For this review, use the dimensioned drawing (mm, ordinates from the lowest corner) and the shaded views. A direction names the side the tool comes from. Coordinates: 2 decimals unless noted, no trailing zeros. Write each loop counter-clockwise with the first axis right and the second up, starting at its lowest first coordinate (ties: lowest second). Pieces come first, ordered by that corner, then holes. Notation, with made-up numbers: (-28.5, 55.25) - (-6.5, 55.25) arc R25 cw to (-6.5, 71.25) - close; hole circle Ø9 at (44, 10.25). An arc over 180 degrees is marked (long way). Answer as a JSON object with one key per item and string values.
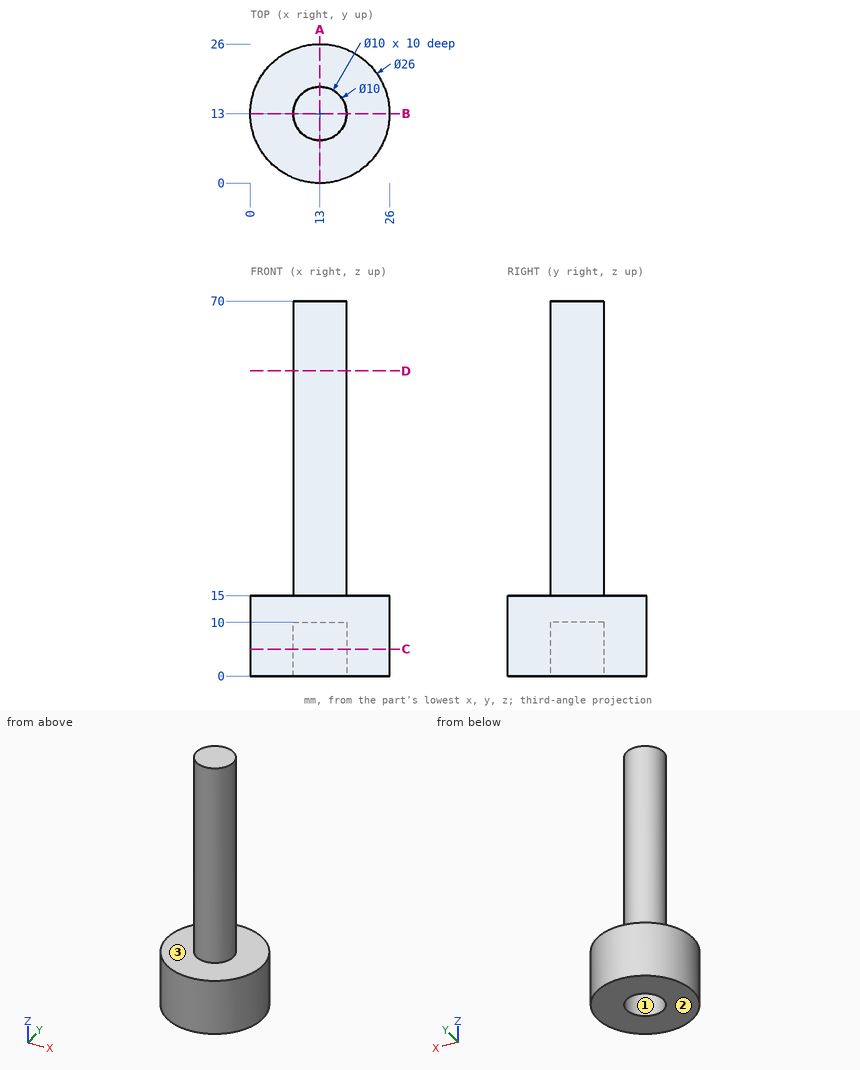
(1) Take a section at C-C, the plane z = 5. Write out the cut boundary in (x, y), and give its area (3 significant figures).
Solved:
{"outline": "circle Ø26 at (13, 13); hole circle Ø10 at (13, 13)", "area": "452 mm^2"}
(2) Take a section at D-D, the plane z = 57. Write out the cut boundary in (x, y), and give its area (3 significant figures).
Solved:
{"outline": "circle Ø10 at (13, 13)", "area": "78.5 mm^2"}
(3) To check wall thickness, follow line 1 (Y direction, x = 13, z = 5.75); line 2 (Z direction, x = 22, y = 4.75); line 3 (Y direction, x = 12.75, z = 16.5). State the ranges of each line that lie inside material, in increasing order. Write a range as from..to.
Solved:
{"line 1": "y = 0..8, 18..26", "line 2": "z = 0..15", "line 3": "y = 8.01..17.99"}
(4) Take a section at A-A, the plane x = 13. Write out the cut boundary in (y, z), and give its area (3 significant figures).
Solved:
{"outline": "(0, 0) - (8, 0) - (8, 10) - (18, 10) - (18, 0) - (26, 0) - (26, 15) - (18, 15) - (18, 70) - (8, 70) - (8, 15) - (0, 15) - close", "area": "840 mm^2"}
(5) Tool access review of the marked faces 1, 2 and 3: name each direction out of +Z, -Z, +X, -X, +Y, -Y from which nothing blocks a thin tool from reaching the whole face with its end or side.
Solved:
{"face 1": "-Z", "face 2": "-Z, +X, -X, +Y, -Y", "face 3": "+Z"}
(6) For pin 1 (8 mm diameter, centred on x = 13.5, y = 12.5, fed in from -Z); pin 2 (5 mm diameter, centred on x = 9.5, z = 24.5, fed in from +Y); pin 3 (1 mm diameter, centred on x = 6.5, y = 12, fed in from +Z), all flat-tipped, find the tip position at first contact; note any pin that passes through.
Solved:
{"pin 1": "stops at z = 10", "pin 2": "stops at y = 17.9", "pin 3": "stops at z = 15"}
